from build123d import *

# Parameters (mm, degrees)
F0_W        = 127
F0_H        = 76.2
F1_DEPTH    = 3.81
F2_R        = 2.813188
F3_DEPTH    = 25.4
F4_W        = 20.256868
F4_H        = 16.464486
F5_DEPTH    = 101.6
F6_W        = 127
F6_H        = 76.2
F6_W_2      = 20.256868
F6_H_2      = 16.464486
F6_R        = 2.813188
F1_FACE_W   = 127
F1_FACE_H   = 76.2
F1_FACE_W_2 = 20.256868
F1_FACE_H_2 = 16.464486
F1_FACE_R   = 2.813188
F7_DEPTH    = 25.4


with BuildPart() as f1:
    # F0 (on Front) → F1 (new body, symmetric)
    with BuildSketch(Plane.XZ):
        Rectangle(F0_W, F0_H)
    extrude(amount=F1_DEPTH, both=True)

    # F2 (on face) → F3 (cut)
    with BuildSketch(Plane.XZ.offset(3.81)):
        with Locations((-38.201306, 17.990688)):
            Circle(F2_R)
    extrude(amount=-F3_DEPTH, mode=Mode.SUBTRACT)

    # F4 (on face) → F5 (cut)
    with BuildSketch(Plane.XZ.offset(3.81)):
        with Locations((-39.635011, -19.933127)):
            Rectangle(F4_W, F4_H)
    extrude(amount=-F5_DEPTH, mode=Mode.SUBTRACT)

    # F6 (on face) + F1_face (on face) → F7 (join)
    with BuildSketch(Plane.XZ.offset(3.81)):
        with BuildLine():
            ThreePointArc((-14.394957, 8.691607), (-8.89384, 14.36516), (-3.220287, 8.864043))
            Line((-3.220287, 8.864043), (-0.426287, 8.864043))
            Line((-0.426287, 8.864043), (-0.426287, 10.68467))
            Line((-0.426287, 10.68467), (-1.648593, 10.68467))
            ThreePointArc((-1.648593, 10.68467), (-8.896568, 16.185919), (-16.01037, 10.512235))
            Line((-16.01037, 10.512235), (-17.188957, 10.512235))
            Line((-17.188957, 10.512235), (-17.188957, 8.691607))
            Line((-17.188957, 8.691607), (-14.394957, 8.691607))
        make_face()
        Rectangle(F6_W, F6_H)
        with Locations((-39.635011, -19.933127)):
            Rectangle(F6_W_2, F6_H_2, mode=Mode.SUBTRACT)
        with Locations((-38.201306, 17.990688)):
            Circle(F6_R, mode=Mode.SUBTRACT)
        with BuildLine():
            Line((-0.426287, 8.864043), (-3.220287, 8.864043))
            ThreePointArc((-3.220287, 8.864043), (-8.89384, 14.36516), (-14.394957, 8.691607))
            Line((-14.394957, 8.691607), (-17.188957, 8.691607))
            Line((-17.188957, 8.691607), (-17.188957, 10.512235))
            Line((-17.188957, 10.512235), (-16.01037, 10.512235))
            ThreePointArc((-16.01037, 10.512235), (-8.896568, 16.185919), (-1.648593, 10.68467))
            Line((-1.648593, 10.68467), (-0.426287, 10.68467))
            Line((-0.426287, 10.68467), (-0.426287, 8.864043))
        make_face(mode=Mode.SUBTRACT)
    with BuildSketch(Plane.XZ.offset(3.81)):
        Rectangle(F1_FACE_W, F1_FACE_H)
        with Locations((-39.635011, -19.933127)):
            Rectangle(F1_FACE_W_2, F1_FACE_H_2, mode=Mode.SUBTRACT)
        with Locations((-38.201306, 17.990688)):
            Circle(F1_FACE_R, mode=Mode.SUBTRACT)
    extrude(amount=F7_DEPTH)


solid = f1.part
Input: part model. Units: mm. Frame: model coordinates. A direction names the side the tool comes from. Give positions to 0.01 mm unless a question says otherwise; leave off trailing zeros. Loops run counter-clockwise (first coordinate to the right, second up) from the corner with the lowest first, then second, coordinate; pieces in that order, holes last. Notation, with made-up numbers: (-30.5, 20.5) -> (5.5, 20.5) arc R21 cw to (5.5, 58.5) -> close; hole circle Ø4 at (6.5, -4.75). An arc over 180 degrees is marked (long way). Answer as a JSON object with one key per item and string values. Group by question number.
Item 1: Cut plane B-B, the plane x = -43. Return the cut outline in (y, z).
Item 2: Cut plane A-A, the plane z = -25.5. Return the cut outline in (x, y).
Item 3: Reachability of faces 1 (the flat face through (-49.763, -12, -20)), 2 (the flat face through (-1, -12, -38.1)) from +Z, -Z, +X, -X, +Y, -Y: full face, straight path, thin tool, end or side. Return the list, or none.
Item 4: Pin query (flat end, axial travel): P1, Ø3.5, axis at x = -38.2, z = 17.99, coming from the -Y side. Return the tip coordinate at first contact, or that it passes through.
Item 5: Line query: probe 1 along Z at (x, y) = (-33.5, -1.5); probe 2 along X at (y, z) = (-1.5, -22.5); probe 3 along X at (y, z) = (-25.5, 18). Output: solid intervals per line, ascending.
Item 6: Pull-direction query (X, two-part tool) for faces 3 (the flat face through (-1, 3.81, 1)), 4 (the flat face through (-29.507, -12, -20)), 5 (the flat face through (63.5, -12, -1)), 6 (the flat face through (-63.5, -12, -1)); classes: released by +X, released by -X, zero draft, split by the parting line, or undercut.
Item 7: Cut plane C-C, the plane y = -23.5. Return the cut outline in (x, z), and give its area (3 significant figures).
Checks:
{
 "1": {"outline": "(-29.21, -38.1) -> (3.81, -38.1) -> (3.81, -28.17) -> (-29.21, -28.17) -> close; (-29.21, -11.7) -> (3.81, -11.7) -> (3.81, 38.1) -> (-29.21, 38.1) -> close"},
 "2": {"outline": "(-63.5, -29.21) -> (-49.76, -29.21) -> (-49.76, 3.81) -> (-63.5, 3.81) -> close; (-29.51, -29.21) -> (63.5, -29.21) -> (63.5, 3.81) -> (-29.51, 3.81) -> close"},
 "3": {"face 1": "+Y, -Y", "face 2": "-Z, +X, -X, +Y, -Y"},
 "4": {"P1": "passes through"},
 "5": {"probe 1": "z = -38.1 to -28.17, -11.7 to 38.1", "probe 2": "x = -63.5 to -49.76, -29.51 to 63.5", "probe 3": "x = -63.5 to -41.01, -35.39 to 63.5"},
 "6": {"face 3": "zero draft", "face 4": "undercut", "face 5": "released by +X", "face 6": "released by -X"},
 "7": {"outline": "(-63.5, -38.1) -> (63.5, -38.1) -> (63.5, 38.1) -> (-63.5, 38.1) -> close; hole (-49.76, -28.17) -> (-29.51, -28.17) -> (-29.51, -11.7) -> (-49.76, -11.7) -> close; hole circle Ø5.63 at (-38.2, 17.99)", "area": "9,320 mm²"}
}
